from build123d import *
from build123d.topology import SkipClean

# Parameters (mm, degrees)
SKETCH1_R           = 1.875
SKETCH1_R_2         = 1.5
BOSS_EXTRUDE1_DEPTH = 3
BOSS_EXTRUDE2_START = 20
SKETCH3_W           = 13
SKETCH3_H           = 8
SKETCH3_R           = 1.5
BOSS_EXTRUDE2_DEPTH = 20
FILLET1_R           = 2


with BuildPart() as part:
    # Sketch1 → Boss-Extrude1 (new body)
    with BuildSketch(Plane(origin=(0, 0, 0), x_dir=(1, 0, 0), z_dir=(0, 1, 0))):
        with BuildLine():
            Line((-10, -4), (10, -4))
            ThreePointArc((10, -4), (14, 0), (10, 4))
            Line((10, 4), (-10, 4))
            ThreePointArc((-10, 4), (-14, 0), (-10, -4))
        make_face()
        with Locations(Location((-10, 0, 0), (0, 0, 270))):
            Circle(SKETCH1_R, mode=Mode.SUBTRACT)
        with Locations(Location((10, 0, 0), (0, 0, 270))):
            Circle(SKETCH1_R, mode=Mode.SUBTRACT)
        with Locations(Location((0, 0, 0), (0, 0, 270))):
            Circle(SKETCH1_R_2, mode=Mode.SUBTRACT)
    extrude(amount=BOSS_EXTRUDE1_DEPTH)

    # Sketch3 → Boss-Extrude2 (add)
    with SkipClean():  # the faces are left unmerged after this step: merging them gives an invalid solid
        with BuildSketch(Plane.XZ.offset(BOSS_EXTRUDE2_START)):
            Rectangle(SKETCH3_W, SKETCH3_H)
            with Locations(Location((0, 0, 0), (0, 0, 270))):
                Circle(SKETCH3_R, mode=Mode.SUBTRACT)
        extrude(amount=-BOSS_EXTRUDE2_DEPTH)

    # Fillet1
    # the kernel refuses this fillet: 2 mm, written as the material it takes off along each edge
    with BuildSketch(Plane(origin=(6.5, -25, -4), x_dir=(0, 0, 1), z_dir=(0, 1, 0)), Plane(origin=(6.5, -25, 4), x_dir=(-1, 0, 0), z_dir=(0, 1, 0))) as fillet1_piece_1:
        with BuildLine():
            CenterArc((FILLET1_R, -FILLET1_R), FILLET1_R, 90, 90)
            Line((0, -FILLET1_R), (0, 0))
            Line((0, 0), (FILLET1_R, 0))
        make_face()
    extrude(amount=25, mode=Mode.SUBTRACT)
    with BuildSketch(Plane(origin=(-6.5, -25, 4), x_dir=(1, 0, 0), z_dir=(0, 1, 0)), Plane(origin=(-6.5, -25, -4), x_dir=(0, 0, 1), z_dir=(0, 1, 0))) as fillet1_piece_2:
        with BuildLine():
            CenterArc((FILLET1_R, FILLET1_R), FILLET1_R, 180, 90)
            Line((0, FILLET1_R), (0, 0))
            Line((0, 0), (FILLET1_R, 0))
        make_face()
    extrude(amount=25, mode=Mode.SUBTRACT)


solid = part.part
Build history of the part. All positions in model axes, mm. A direction names the side the tool comes from. Coordinates: 2 decimals unless noted, no trailing zeros. Order: outer loops, then holes, each group sorted by start corner. A loop starts at its lowest first (then second) coordinate and runs counter-clockwise, first axis right, second up. Notation, with made-up numbers: M 82,-21.75 L 133,-21.75 A19 cw 133,-16.75 Z; hole C 9,65 d7. An arc over 180 degrees is marked long. One line per question, with ' | ' between items. Start each with the question number.
Q1. Flat gauge pins, fed straight in: pin 1 Ø2.5 at (x, z) = (-11, 1.5) entering from -Y; pin 2 Ø4.5 at (x, z) = (-10, 0) entering from +Y; pin 3 Ø3 at (y, z) = (-13.5, -1.5) entering from +X; pin 4 Ø4.5 at (y, z) = (-13, -0.5) entering from -X. Where does each tip first touch, or does it go through?
Q2. Saw through at C-C (x = 0). List the corners of the cut face in (y, z).
Q3. Probe L1, parallel to X at y = 2.4, z = 0 (3 decimals); L2, parallel to Z at x = 0, y = -14.75; L3, parallel to X at y = -18.25, z = 0. List the from-to ranges inside material, lowest first. Write a range as from..to.
Q4. 3-axis set-ups, long thin cutter, end or side, ignore diameter. For faces 1 (the face through (5.93, -10.14, -3.4)), 2 (the face through (-5.93, -10.14, 3.4)), 3 (the face through (5.9, -10.14, 3.43)), 4 (the face through (6.5, -10, 0)): which of +Z, -Z, +X, -X, +Y, -Y reach the whole face in a straight line?
Q5. Saw through at D-D (z = -2.5). List the corners of the cut face in (x, y), then the cut area to 3 significant figures.
Q6. Saw through at B-B (y = -1). List the corners of the cut face in (x, z), then the cut area to 3 significant figures.
Q7. Saw through at A-A (z = 0). List the corners of the cut face in (x, y) (3 decimals).
Q8. Two-plate mould, pull along X, no slides. Class faces 5 (the face through (-5.9, -10.14, -3.43)), 6 (the face through (8, 0, 1)), 7 (the face through (-11.83, 1.48, -0.41)): +X half, -X half, draft (parallel to the pull), parting line (faces both ways), or undercut.
Check values:
1) pin 1: stops at y = 0 | pin 2: stops at y = 3 | pin 3: stops at x = 6.5 | pin 4: stops at x = -6.5
2) outline: M -20,-4 L 3,-4 L 3,-1.5 L -20,-1.5 Z; M -20,1.5 L 3,1.5 L 3,4 L -20,4 Z
3) L1: x = -14..-11.875, -8.125..-1.5, 1.5..8.125, 11.875..14 | L2: z = -4..-1.5, 1.5..4 | L3: x = -6.5..-1.5, 1.5..6.5
4) face 1: -Z, +X, -Y | face 2: +Z, -X, -Y | face 3: +Z, +X, -Y | face 4: +Z, -Z, +X, -Y
5) outline: M -13.12,0 L -6.44,0 L -6.44,-20 L 6.44,-20 L 6.44,0 L 13.12,0 L 13.12,3 L -13.12,3 Z | area: 336 mm2
6) outline: M -6.5,-2 A2 ccw -4.5,-4 L 4.5,-4 A2 ccw 6.5,-2 L 6.5,2 A2 ccw 4.5,4 L -4.5,4 A2 ccw -6.5,2 Z; hole C 0,0 d3 | area: 93.5 mm2
7) outline: M -14,0 L -11.875,0 L -11.875,3 L -14,3 Z; M -8.125,0 L -6.5,0 L -6.5,-20 L -1.5,-20 L -1.5,3 L -8.125,3 Z; M 1.5,-20 L 6.5,-20 L 6.5,0 L 8.125,0 L 8.125,3 L 1.5,3 Z; M 11.875,0 L 14,0 L 14,3 L 11.875,3 Z
8) face 5: -X half | face 6: draft | face 7: undercut
